from build123d import *

# Parameters (mm, degrees)
CHAMFER_1_SIZE           = 1
SKETCH_2_W               = 19
SKETCH_2_H               = 4
CUT_EXTRUDE_1_DEPTH      = 4
CUT_EXTRUDE_3_DEPTH      = 255.770484947
PATTERN_CIRCULAR_1_COUNT = 2
PATTERN_CIRCULAR_1_ANGLE = 18
F_1_THE_OTHER_WAY_COUNT  = 2
F_1_THE_OTHER_WAY_ANGLE  = 18


with BuildPart() as part:
    # 草图1 → 旋转1 (revolve)
    with BuildSketch(Plane.XY, mode=Mode.PRIVATE) as revolve_1_sk:
        Polygon((-264, 0), (-264, 6), (-219, 6), (-219, 7), (-39, 7), (-39, 9.5), (-16, 9.5), (-16, 14), (-10, 14), (-10, 9.5), (0, 9.5), (0, 0), align=None)
    revolve(revolve_1_sk.sketch.rotate(Axis((0, 0, 0), (-1, 0, 0)), 90), axis=Axis((0, 0, 0), (-1, 0, 0)))

    # 倒角1
    chamfer_1_edges = [part.edges().sort_by_distance(p)[0] for p in [
        (-264, 0, 6),
    ]]
    chamfer(chamfer_1_edges, length=CHAMFER_1_SIZE)

    # 草图2 → 切除-拉伸-薄壁1 (cut)
    with BuildSketch(Plane(origin=(0, 0, 0), x_dir=(0, 0, -1), z_dir=(1, 0, 0))):
        Rectangle(SKETCH_2_W, SKETCH_2_H)
    extrude(amount=-CUT_EXTRUDE_1_DEPTH, mode=Mode.SUBTRACT)

    # 草图4 → 切除-拉伸3 (cut, symmetric)
    with BuildSketch(Plane(origin=(-10, 0, 0), x_dir=(0, 0, -1), z_dir=(1, 0, 0))):
        Polygon((0, -89.785980761), (0, -14), (0, -10.3), (-4.326237921, -13.314791228), (-66.504055872, -56.644155807), (-134.109197976, -192.304040375), (-67.605142103, -225.445865329), align=None)
    cut_extrude_3 = extrude(amount=CUT_EXTRUDE_3_DEPTH, both=True, mode=Mode.SUBTRACT)

    # 阵列(圆周)1: 切除-拉伸3 ×2 about axis
    pattern_circular_1_axis = Axis((0, 0, 0), (1, 0, 0))
    for i in range(1, PATTERN_CIRCULAR_1_COUNT):
        add(cut_extrude_3.rotate(pattern_circular_1_axis, i * PATTERN_CIRCULAR_1_ANGLE / (PATTERN_CIRCULAR_1_COUNT - 1)), mode=Mode.SUBTRACT)

    # 1 the other way: 切除-拉伸3 ×2 about axis
    f_1_the_other_way_axis = Axis((0, 0, 0), (-1, 0, 0))
    for i in range(1, F_1_THE_OTHER_WAY_COUNT):
        add(cut_extrude_3.rotate(f_1_the_other_way_axis, i * F_1_THE_OTHER_WAY_ANGLE / (F_1_THE_OTHER_WAY_COUNT - 1)), mode=Mode.SUBTRACT)


solid = part.part
Verification items for the finished model (mm, model axes). A direction names the side the tool comes from. Give positions to 0.01 mm unless a question says otherwise; leave off trailing zeros. Write each loop counter-clockwise with the first axis right and the second up, starting at its lowest first coordinate (ties: lowest second). Pieces come first, ordered by that corner, then holes. Notation, with made-up numbers: M 74.5,26.25 L 128.5,26.25 A13 cw 128.5,33.25 Z; hole C 65.25,-28 d9. An arc over 180 degrees is marked long. Put each result on its own line as item: value. Start each with the question number.
1. Set-up check for faces 1 (the face through (-264, 0, 0)), 2 (the face through (-240.692, -1.802, -5.723)): record each of +Z, -Z, +X, -X, +Y, -Y from which the full face is reachable in a straight line by a thin tool's end or side.
2. Scan lines: line 1 along X through (y, z) = (-11.75, -0.5); line 2 along X through (y, z) = (5.25, -7); line 3 along Z through (x, y) = (-167, 5.5). Record each from-to range of solid material in increasing order. Write a range as [from, to].
3. Draft check along Z on faces 3 (the face through (-12.96, -10.55, 5.67)), 4 (the face through (-10, 9.1, 3.3)), 5 (the face through (-4.93, -2.854, -9.061)), 6 (the face through (-12.958, -11.869, -1.614)). Enter one of: +Z half, -Z half, draft (parallel to the pull), parting line (faces both ways), or undercut.
4. Go/stop test with flat-tipped pins: pin 1 Ø3 at (x, y) = (-144.5, 2) entering from +Z; pin 2 Ø10 at (x, z) = (-110.5, 1.5) entering from +Y; pin 3 Ø8 at (x, y) = (-111, -7.5) entering from -Z; pin 4 Ø10 at (y, z) = (0.5, 2.5) entering from +X. Record where each tip stops, or that it passes through.
5. Section check A-A (x = -27). Record the cut outline in (y, z).
6. Section check B-B (x = -78). Record the cut outline in (y, z).
Answer list:
1. face 1: +Z, -Z, -X, +Y, -Y
1. face 2: -X
2. line 1: [-16, -10]
2. line 2: [-39, 0]
2. line 3: [-4.33, 4.33]
3. face 3: undercut
3. face 4: draft
3. face 5: parting line
3. face 6: undercut
4. pin 1: z = 6.98
4. pin 2: y = 7
4. pin 3: z = -6.06
4. pin 4: x = 0
5. outline: C 0,0 d19
6. outline: C 0,0 d14
